```python
from build123d import *

# Parameters (mm, degrees)
SKETCH_1_W             = 110
SKETCH_1_H             = 85
EXTRUDE_1_DEPTH        = 6
SKETCH_2_R             = 36
CUT_EXTRUDE_1_DEPTH    = 10
CUT_EXTRUDE_2_DEPTH    = 10
HOLE_WIZARD_M6_1_D     = 5
HOLE_WIZARD_M6_1_DEPTH = 15
HOLE_WIZARD_M6_1_TIP   = 1.502151548


with BuildPart() as part:
    # 草图1 → 凸台-拉伸1 (new body)
    with BuildSketch(Plane(origin=(0, 0, 0), x_dir=(1, 0, 0), z_dir=(0, 1, 0))):
        Rectangle(SKETCH_1_W, SKETCH_1_H)
    extrude(amount=EXTRUDE_1_DEPTH)

    # 草图2 → 切除-拉伸1 (cut)
    with BuildSketch(Plane(origin=(0, 6, 0), x_dir=(1, 0, 0), z_dir=(0, 1, 0))):
        Circle(SKETCH_2_R)
    extrude(amount=-CUT_EXTRUDE_1_DEPTH, mode=Mode.SUBTRACT)

    # 草图3 → 切除-拉伸2 (cut)
    with BuildSketch(Plane(origin=(0, 6, 0), x_dir=(1, 0, 0), z_dir=(0, 1, 0))):
        with BuildLine():
            Line((-45.5, 36), (-45.5, 26))
            ThreePointArc((-45.5, 26), (-49, 22.5), (-52.5, 26))
            Line((-52.5, 26), (-52.5, 36))
            ThreePointArc((-52.5, 36), (-49, 39.5), (-45.5, 36))
        make_face()
        with BuildLine():
            Line((45.5, 36), (45.5, 26))
            ThreePointArc((45.5, 26), (49, 22.5), (52.5, 26))
            Line((52.5, 26), (52.5, 36))
            ThreePointArc((52.5, 36), (49, 39.5), (45.5, 36))
        make_face()
        with BuildLine():
            Line((-45.5, -36), (-45.5, -26))
            ThreePointArc((-45.5, -26), (-49, -22.5), (-52.5, -26))
            Line((-52.5, -26), (-52.5, -36))
            ThreePointArc((-52.5, -36), (-49, -39.5), (-45.5, -36))
        make_face()
        with BuildLine():
            Line((45.5, -36), (45.5, -26))
            ThreePointArc((45.5, -26), (49, -22.5), (52.5, -26))
            Line((52.5, -26), (52.5, -36))
            ThreePointArc((52.5, -36), (49, -39.5), (45.5, -36))
        make_face()
    extrude(amount=-CUT_EXTRUDE_2_DEPTH, mode=Mode.SUBTRACT)

    # M6 螺纹孔1
    with Locations(Plane(origin=(-31.819805153, 6, -31.819805153), x_dir=(0, 0, 1), z_dir=(0, 1, 0))):
        with Locations((0, 0), (0, 63.639610306), (63.639610306, 63.639610306), (63.639610306, 0)):
            Hole(HOLE_WIZARD_M6_1_D / 2, depth=HOLE_WIZARD_M6_1_DEPTH)
            with Locations((0, 0, -(HOLE_WIZARD_M6_1_DEPTH + HOLE_WIZARD_M6_1_TIP / 2))):  # 118° drill point
                Cone(0, HOLE_WIZARD_M6_1_D / 2, HOLE_WIZARD_M6_1_TIP, mode=Mode.SUBTRACT)


solid = part.part
```
Input: part model. Units: mm. Frame: model coordinates. A direction names the side the tool comes from. Give positions to 0.01 mm unless a question says otherwise; leave off trailing zeros. Write each loop counter-clockwise with the first axis right and the second up, starting at its lowest first coordinate (ties: lowest second). Pieces come first, ordered by that corner, then holes. Notation, with made-up numbers: (63, 77) - (72, 77) arc R18 ccw to (72, 90) - close; hole circle Ø2 at (18, -19.5). An arc over 180 degrees is marked (long way). Write item = value, one per line. Start each with the question number.
1. Mould query, pull axis X, two halves, no side actions, for faces 3 (the flat face through (-37, 0, -1)), 4 (the flat face through (52.5, 3, -31)), 5 (the flat face through (-55, 3, 1)). Classes: released by +X, released by -X, zero draft, split by the parting line, or undercut.
2. Section query B-B, the plane z = 24. Output: boundary loops of the cut face in (x, y), then the cut area to 3 significant figures.
3. Access query for faces 1 (the flat face through (55, 3, 1)), 2 (the flat face through (52.5, 3, 31)). Directions: +Z, -Z, +X, -X, +Y, -Y. A direction counts if a zero-diameter tool reaches every point of the face in a straight line with its end or side. Return the directions, or none.
4. Section query A-A, the plane x = 0. Output: boundary loops of the cut face in (y, z), then the cut area to 3 significant figures.
5. Ray query, L1, parallel to Z at x = 0, y = 4.3; L2, parallel to Z at x = -32.5, y = 4.75; L3, parallel to Z at x = -33, y = 4.05. Return the intervals inside material, ascending.
6. Section query C-C, the plane z = 4. Output: boundary loops of the cut face in (x, y).
7. Section query D-D, the plane x = 49. Output: boundary loops of the cut face in (y, z), then the cut area to 3 significant figures.
Check sheet entries:
q1.face_3 = zero draft
q1.face_4 = undercut
q1.face_5 = released by -X
q2.outline = (-55, 0) - (-51.87, 0) - (-51.87, 6) - (-55, 6) - close; (-46.13, 0) - (-26.83, 0) - (-26.83, 6) - (-46.13, 6) - close; (26.83, 0) - (46.13, 0) - (46.13, 6) - (26.83, 6) - close; (51.87, 0) - (55, 0) - (55, 6) - (51.87, 6) - close
q2.area = 269 mm2
q3.face_1 = +Z, -Z, +X, +Y, -Y
q3.face_2 = +Y, -Y
q4.outline = (0, -42.5) - (6, -42.5) - (6, -36) - (0, -36) - close; (0, 36) - (6, 36) - (6, 42.5) - (0, 42.5) - close
q4.area = 78.0 mm2
q5.L1 = -42.5 to -36, 36 to 42.5
q5.L2 = -42.5 to -34.23, -29.41 to -15.48, 15.48 to 29.41, 34.23 to 42.5
q5.L3 = -42.5 to -34.02, -29.62 to -14.39, 14.39 to 29.62, 34.02 to 42.5
q6.outline = (-55, 0) - (-35.78, 0) - (-35.78, 6) - (-55, 6) - close; (35.78, 0) - (55, 0) - (55, 6) - (35.78, 6) - close
q7.outline = (0, -42.5) - (6, -42.5) - (6, -39.5) - (0, -39.5) - close; (0, -22.5) - (6, -22.5) - (6, 22.5) - (0, 22.5) - close; (0, 39.5) - (6, 39.5) - (6, 42.5) - (0, 42.5) - close
q7.area = 306 mm2
